Can you work these out from the model? Positions are in its coordinate system, mm. A direction names the side the tool comes from. Round coordinates to 2 decimals unless told otherwise and drop trailing zeros. Loops run counter-clockwise (first coordinate to the right, second up) from the corner with the lowest first, then second, coordinate; pieces in that order, holes last.
from build123d import *

# Parameters (mm, degrees)
SKETCH1_R           = 4.05
SKETCH1_R_2         = 4
BOSS_EXTRUDE1_DEPTH = 25.4


with BuildPart() as part:
    # Sketch1 → Boss-Extrude1 (new body)
    with BuildSketch(Plane(origin=(0, 0, 0), x_dir=(1, 0, 0), z_dir=(0, 1, 0))):
        with BuildLine():
            Line((35.095585876, 75.150873895), (-72.841125884, 75.150873895))
            ThreePointArc((-72.841125884, 75.150873895), (-85.568525883, 62.423473896), (-72.841125884, 49.696073896))
            Line((-72.841125884, 49.696073896), (38.270585876, 49.696073896))
            Line((38.270585876, 49.696073896), (63.158100717, 49.696073896))
            ThreePointArc((63.158100717, 49.696073896), (63.742381743, 49.723011689), (64.321705528, 49.803596516))
            ThreePointArc((64.321705528, 49.803596516), (80.546596989, 54.618688797), (95.424112169, 62.686635169))
            ThreePointArc((95.424112169, 62.686635169), (95.890738024, 63.039296868), (96.322934996, 63.433398048))
            Line((96.322934996, 63.433398048), (110.746065504, 77.856528557))
            ThreePointArc((110.746065504, 77.856528557), (111.43431899, 81.316612485), (108.501001474, 83.276592587))
            Line((108.501001474, 83.276592587), (107.323802413, 83.276592587))
            ThreePointArc((107.323802413, 83.276592587), (104.646034573, 84.74566633), (104.44627519, 87.793405568))
            Line((104.44627519, 87.793405568), (147.384290582, 179.874276731))
            ThreePointArc((147.384290582, 179.874276731), (141.241433611, 196.75163755), (124.364072791, 190.608780579))
            Line((124.364072791, 190.608780579), (76.090158478, 87.085037255))
            ThreePointArc((76.090158478, 87.085037255), (74.19673791, 85.408214933), (71.67884134, 85.646901766))
            ThreePointArc((71.67884134, 85.646901766), (69.496098635, 87.053305606), (67.524885923, 88.743470663))
            ThreePointArc((67.524885923, 88.743470663), (46.789721423, 92.732243213), (35.095585876, 75.150873895))
        make_face()
        with Locations((54.158874116, 75.150873895)):
            Circle(SKETCH1_R, mode=Mode.SUBTRACT)
        with Locations((135.874181687, 185.241528655)):
            Circle(SKETCH1_R_2, mode=Mode.SUBTRACT)
    extrude(amount=BOSS_EXTRUDE1_DEPTH)


solid = part.part
(1) For faces 4 (the flat face through (125.615, 12.522, -133.189)), 5 (the flat face through (-18, 13, -75.151)), 6 (the cylindrical face through (-85.565, 12.522, -62.703)), which set-ups out of +Z, -Z, +X, -X, +Y, -Y let a thin tool reach every point of the face, with its end or its side?
Worked answers:
face 4: +X, +Y, -Y
face 5: -Z, -X, +Y, -Y
face 6: -X, +Y, -Y
(2) If we section it at A-A, the plane y = 12.25: List the corners of the cut face in (x, z) for me (3 decimals).
Worked answers:
outline: (-72.841, -75.151) - (35.096, -75.151) arc R19.063 ccw to (67.525, -88.743) arc R19.05 cw to (71.679, -85.647) arc R3.175 cw to (76.09, -87.085) - (124.364, -190.609) arc R12.7 ccw to (147.384, -179.874) - (104.446, -87.793) arc R3.175 cw to (107.324, -83.277) - (108.501, -83.277) arc R3.175 ccw to (110.746, -77.857) - (96.323, -63.433) arc R6.35 ccw to (95.424, -62.687) arc R81.353 ccw to (64.322, -49.804) arc R6.35 ccw to (63.158, -49.696) - (-72.841, -49.696) arc R12.727 ccw to start; hole circle Ø8.1 at (54.159, -75.151); hole circle Ø8 at (135.874, -185.242)
(3) If we section it at C-C, the plane z = -140.5: List the corners of the cut face in (x, y) for me.
Worked answers:
outline: (101, 0) - (129.02, 0) - (129.02, 25.4) - (101, 25.4) - close
(4) If I drill on line 1 (Z direction, x = -33.5, y = 15.25); line 2 (Z direction, x = 105, y = 23.5); line 3 (X direction, y = 16.5, z = -191), over which ranges is the centre line in solid material (lowest first)?
Worked answers:
line 1: z = -75.15 to -49.7
line 2: z = -149.08 to -88.98, -84.29 to -72.11
line 3: x = 124.55 to 147.19
(5) If we mould it in two halves opening along Z, with no side actions, what happens to faces 1 (the cylindrical face through (47.08, 12.52, -92.85)), 2 (the cylindrical face through (111.454, 12.522, -81.268)), 3 (the flat face through (48, 25.4, -91))? For each: released by +Z, released by -Z, zero draft, split by the parting line, or undercut.
Worked answers:
face 1: released by -Z
face 2: undercut
face 3: zero draft
(6) If we section it at B-B, the plane x = -46.5: List the corners of the cut face in (y, z) for me.
Worked answers:
outline: (0, -75.15) - (25.4, -75.15) - (25.4, -49.7) - (0, -49.7) - close
(7) Will these pins go through, and if not, where does the flat tip stop? P1, Ø8, axis at y = 11.5, z = -67.5, coming from the -X side; P2, Ø12, axis at y = 17.5, z = -97.5, coming from the -X side; P3, Ø3, axis at y = 6, z = -171.5, coming from the -X side.
Worked answers:
P1: stops at x = -85.52
P2: stops at x = 44.36
P3: stops at x = 114.75
